CAD build for the part. Positions are in the model's coordinates, mm. Coordinates: 2 decimals unless noted, no trailing zeros. Write each loop counter-clockwise with the first axis right and the second up, starting at its lowest first coordinate (ties: lowest second). Pieces come first, ordered by that corner, then holes. Notation, with made-up numbers: (-22.5, -19.75) - (31.5, -19.75) arc R26 ccw to (31.5, 6.25) - close; hole circle Ø7 at (-15, -1.5). An arc over 180 degrees is marked (long way). One line per question, with ' | ' between items. Start each with the question number.
1. Two-plate mould, pull along Z, no slides. Class faces 1 (the flat face through (0, 1, 13.5)), 2 (the flat face through (-29, -0.005, 13)), 3 (the cylindrical face through (-30.774, 0.593, 11.876)), 4 (the flat face through (0, 1, -13.5)): +Z half, -Z half, draft (parallel to the pull), parting line (faces both ways), or undercut.
2. Band-saw the part on D-D, the plane x = 19. Write the cut outline in (y, z).
3. Band-saw the part on B-B, the plane x = -20.19. Write the cut outline in (y, z) (3 decimals).
4. Flat gauge pins, fed straight in: P1, Ø2, axis at x = 23.5, z = 4.5, coming from the +Y side; P2, Ø1.8, axis at x = -29.775, z = 11.92, coming from the -Y side; P3, Ø5, axis at x = 10, z = -4.5, coming from the -Y side. Where does each tip first touch, or does it go through?
5. Band-saw the part on C-C, the plane z = -6.18. Write the cut outline in (x, y) (3 decimals), then the cut area to 3 significant figures.
6. Probe line 1 (X direction, y = 0.7, z = 11.92) (3 decimals); line 2 (X direction, y = 0.35, z = 7.75) (3 decimals); line 3 (Y direction, x = 5.5, z = -7.75). List the from-to ranges inside material, lowest first.
7. Band-saw the part on A-A, the plane z = 11.92. Write the cut outline in (x, y) (3 decimals).
from build123d import *

# Parameters (mm, degrees)
SKETCH1_W                = 64.65
SKETCH1_H                = 27
BOSS_EXTRUDE1_DEPTH      = 1.16
FILLET1_R                = 1
SKETCH2_R                = 1
SKETCH2_R_2              = 1.285
CUT_EXTRUDE1_DEPTH       = 2.16
SKETCH3_R                = 1.5
SKETCH3_R_2              = 1
BOSS_EXTRUDE2_DEPTH      = 0.015
BOSS_EXTRUDE2_DEPTH_BACK = 1.165


with BuildPart() as part:
    # Sketch1 → Boss-Extrude1 (new body)
    with BuildSketch(Plane(origin=(0, 0, 0), x_dir=(1, 0, 0), z_dir=(0, 1, 0))):
        Rectangle(SKETCH1_W, SKETCH1_H)
    extrude(amount=BOSS_EXTRUDE1_DEPTH)

    # Fillet1
    fillet1_edges = [part.edges().sort_by_distance(p)[0] for p in [
        (32.325, 0.58, 13.5),
        (-32.325, 0.58, 13.5),
        (-32.325, 0.58, -13.5),
        (32.325, 0.58, -13.5),
    ]]
    fillet(fillet1_edges, radius=FILLET1_R)

    # Sketch2 → Cut-Extrude1 (cut, through all)
    with BuildSketch(Plane(origin=(0, 1.16, 0), x_dir=(1, 0, 0), z_dir=(0, 1, 0))):
        with Locations((-29.775, -11.92)):
            Circle(SKETCH2_R)
        with Locations((-29.775, 10.08)):
            Circle(SKETCH2_R)
        with Locations((-20.19, -7.105)):
            Circle(SKETCH2_R_2)
        with Locations((-20.19, 6.18)):
            Circle(SKETCH2_R_2)
        with Locations((8.845, -7.105)):
            Circle(SKETCH2_R_2)
    extrude(amount=-CUT_EXTRUDE1_DEPTH, mode=Mode.SUBTRACT)

    # Sketch3 → Boss-Extrude2 (add, two sides)
    with BuildSketch(Plane(origin=(0, 1.16, 0), x_dir=(1, 0, 0), z_dir=(0, 1, 0))) as boss_extrude2_sk:
        with Locations((-29.775, -11.92)):
            Circle(SKETCH3_R)
        with Locations((-29.775, -11.92)):
            Circle(SKETCH3_R_2, mode=Mode.SUBTRACT)
        with Locations((-29.775, 10.08)):
            Circle(SKETCH3_R)
        with Locations((-29.775, 10.08)):
            Circle(SKETCH3_R_2, mode=Mode.SUBTRACT)
    extrude(amount=BOSS_EXTRUDE2_DEPTH)
    extrude(boss_extrude2_sk.sketch, amount=-BOSS_EXTRUDE2_DEPTH_BACK)


solid = part.part
Filled in:
1) face 1: +Z half | face 2: draft | face 3: undercut | face 4: -Z half
2) outline: (0, -13.5) - (1.16, -13.5) - (1.16, 13.5) - (0, 13.5) - close
3) outline: (0, -13.5) - (1.16, -13.5) - (1.16, -7.465) - (0, -7.465) - close; (0, -4.895) - (1.16, -4.895) - (1.16, 5.82) - (0, 5.82) - close; (0, 8.39) - (1.16, 8.39) - (1.16, 13.5) - (0, 13.5) - close
4) P1: stops at y = 1.16 | P2: passes through | P3: stops at y = 0
5) outline: (-32.325, 0) - (-21.475, 0) - (-21.475, 1.16) - (-32.325, 1.16) - close; (-18.905, 0) - (32.325, 0) - (32.325, 1.16) - (-18.905, 1.16) - close | area: 72.0 mm²
6) line 1: x = -32.325 to -30.775, -28.775 to 32.325 | line 2: x = -32.325 to -21.301, -19.079 to 7.734, 9.956 to 32.325 | line 3: y = 0 to 1.16
7) outline: (-32.325, 0) - (-31.275, 0) - (-31.275, -0.005) - (-30.775, -0.005) - (-30.775, 1.175) - (-31.275, 1.175) - (-31.275, 1.16) - (-32.325, 1.16) - close; (-28.775, -0.005) - (-28.275, -0.005) - (-28.275, 0) - (32.325, 0) - (32.325, 1.16) - (-28.275, 1.16) - (-28.275, 1.175) - (-28.775, 1.175) - close
